Geometry check sheet. Reference: the model listing, model coordinates, mm. A direction names the side the tool comes from. Round coordinates to 2 decimals unless told otherwise and drop trailing zeros. Write each loop counter-clockwise with the first axis right and the second up, starting at its lowest first coordinate (ties: lowest second). Pieces come first, ordered by that corner, then holes. Notation, with made-up numbers: M 16,-16.75 L 64,-16.75 A24 cw 64,14.25 Z; hole C -23.5,0 d10. An arc over 180 degrees is marked long. Answer in a Markdown table with one row per item. Add a question column.
from build123d import *

# Parameters (mm, degrees)
SKETCH1_R           = 1.524
BOSS_EXTRUDE1_DEPTH = 1.5875
SKETCH2_W           = 24.638
SKETCH2_H           = 17.272
BOSS_EXTRUDE2_DEPTH = 19.05


with BuildPart() as part:
    # Sketch1 → Boss-Extrude1 (new body)
    with BuildSketch(Plane.XY):
        Polygon((-26.924, 25.4), (-26.924, -19.05), (-14.224, -19.05), (-14.224, -25.4), (14.224, -25.4), (14.224, -19.05), (26.924, -19.05), (26.924, 25.4), align=None)
        with Locations((-10.414, -22.225)):
            Circle(SKETCH1_R, mode=Mode.SUBTRACT)
        with Locations((10.414, -22.225)):
            Circle(SKETCH1_R, mode=Mode.SUBTRACT)
        with Locations((-23.749, 22.225)):
            Circle(SKETCH1_R, mode=Mode.SUBTRACT)
        with Locations((23.749, 22.225)):
            Circle(SKETCH1_R, mode=Mode.SUBTRACT)
    extrude(amount=BOSS_EXTRUDE1_DEPTH)

    # Sketch2 → Boss-Extrude2 (add)
    with BuildSketch(Plane.XY.offset(1.5875)):
        with Locations((0, 15.24)):
            Rectangle(SKETCH2_W, SKETCH2_H)
    extrude(amount=BOSS_EXTRUDE2_DEPTH)


solid = part.part
Item 1: Gauge pin test, flat ends, axial feed: pin 1 Ø0.8 at (x, z) = (20.5, 0.5) entering from -Y; pin 2 Ø2 at (x, y) = (20, -8.5) entering from +Z; pin 3 Ø5 at (y, z) = (15.5, 18.5) entering from +X. Record the tip position at first contact, or that the pin passes through.
Item 2: Section check D-D, the plane z = 16.75. Record the boundary of the cut face in (x, y), and give its area (3 significant figures).
Item 3: Access from +Z, -Z, +X, -X, +Y, -Y to the whole of each face (thin tool, end or side, straight path). Record for faces 1 (the flat face through (-21, -19.05, 1)), 2 (the flat face through (0, 23.876, 11)), 3 (the flat face through (20, -19.05, 1)).
Item 4: Mould release check, pull along Y, two halves, no side actions. Record for faces 4 (the flat face through (26.924, 3, 1)), 5 (the cylindrical face through (23.419, 20.737, 0.783)), 6 (the flat face through (0, 25.4, 1)): +Y half, -Y half, draft (parallel to the pull), parting line (faces both ways), or undercut.
Item 5: Section check C-C, the plane y = 11.5. Record the boundary of the cut face in (x, z).
Item 6: Section check A-A, the plane x = 7. Record the boundary of the cut face in (y, z), and give its area (3 significant figures).
Item 7: Scan lines: probe 1 along Y at (x, z) = (-18.5, 1); probe 2 along X at (y, z) = (17.5, 10.75); probe 3 along Y at (x, z) = (6, 14.75). Record each from-to range of solid material in increasing order. Write a range as from..to.
Item 8: Section check B-B, the plane x = -23. Record the boundary of the cut face in (y, z).
Result sheet:
| question | item | result |
|---|---|---|
| 1 | pin 1 | stops at y = -19.05 |
| 1 | pin 2 | stops at z = 1.59 |
| 1 | pin 3 | stops at x = 12.32 |
| 2 | outline | M -12.32,6.6 L 12.32,6.6 L 12.32,23.88 L -12.32,23.88 Z |
| 2 | area | 426 mm^2 |
| 3 | face 1 | +Z, -Z, -X, -Y |
| 3 | face 2 | +Z, +X, -X, +Y |
| 3 | face 3 | +Z, -Z, +X, -Y |
| 4 | face 4 | draft |
| 4 | face 5 | undercut |
| 4 | face 6 | +Y half |
| 5 | outline | M -26.92,0 L 26.92,0 L 26.92,1.59 L 12.32,1.59 L 12.32,20.64 L -12.32,20.64 L -12.32,1.59 L -26.92,1.59 Z |
| 6 | outline | M -25.4,0 L 25.4,0 L 25.4,1.59 L 23.88,1.59 L 23.88,20.64 L 6.6,20.64 L 6.6,1.59 L -25.4,1.59 Z |
| 6 | area | 410 mm^2 |
| 7 | probe 1 | y = -19.05..25.4 |
| 7 | probe 2 | x = -12.32..12.32 |
| 7 | probe 3 | y = 6.6..23.88 |
| 8 | outline | M -19.05,0 L 20.9,0 L 20.9,1.59 L -19.05,1.59 Z; M 23.55,0 L 25.4,0 L 25.4,1.59 L 23.55,1.59 Z |
